```python
from build123d import *

# Parameters (mm, degrees)
F1_DEPTH         = 844.55
F3_D             = 4.7625
F3_DEPTH         = 25.4
F3_CSINK_D       = 9.525
F3_CSINK_ANGLE   = 90
F3_TIP           = 1.4307993491
F3_COPIES2_COUNT = 2


# Not quite as in the source:
# - a pattern or mirror of a feature is missing from the dataset's text; its kind, count and spacing are read off the source's solid


with BuildPart() as f1:
    # F0 (on Front) → F1 (new body, symmetric)
    with BuildSketch(Plane.XZ):
        Polygon((155.575, -103.1875), (155.575, 103.1875), (-155.575, 103.1875), (-155.575, -103.1875), (-152.4, -103.1875), (-152.4, 100.0125), (152.4, 100.0125), (152.4, -103.1875), align=None)
    extrude(amount=F1_DEPTH, both=True)

    # F3
    with Locations(Plane.YZ.offset(155.575)):
        with Locations((-793.75, -52.3875)):
            f3 = CounterSinkHole(F3_D / 2, F3_CSINK_D / 2, depth=F3_DEPTH, counter_sink_angle=F3_CSINK_ANGLE)
            with Locations((0, 0, -(F3_DEPTH + F3_TIP / 2))):  # 118° drill point
                Cone(0, F3_D / 2, F3_TIP, mode=Mode.SUBTRACT)

    # F3_copies: F3 across plane
    add(f3.mirror(Plane(origin=(0, 0, 0), x_dir=(0, 0, -1), z_dir=(-1, 0, 0))), mode=Mode.SUBTRACT)

    # F3_copies1: F3 across plane
    add(f3.mirror(Plane.ZX), mode=Mode.SUBTRACT)

    # F3_copies2: F3 ×2 about axis
    f3_copies2_axis = Axis((0, 0, 0), (0, 0, 1))
    for i in range(1, F3_COPIES2_COUNT):
        add(f3.rotate(f3_copies2_axis, i * 360 / F3_COPIES2_COUNT), mode=Mode.SUBTRACT)


solid = f1.part
```
Could you check a few things on this model? Use its own coordinates, in mm. A direction names the side the tool comes from. Round coordinates to 2 decimals unless told otherwise and drop trailing zeros. Loops run counter-clockwise (first coordinate to the right, second up) from the corner with the lowest first, then second, coordinate; pieces in that order, holes last. Notation, with made-up numbers: (12, 78) - (63, 78) arc R13 cw to (63, 97) - close; hole circle Ø9 at (-5, 86.25). An arc over 180 degrees is marked (long way). Answer in a Markdown table with one row per item. Add a question column.
(1) For faces 1 (the face through (-2, -12, 100.012)), 2 (the face through (2, -12, 103.188)), which set-ups out of +Z, -Z, +X, -X, +Y, -Y let a thin tool reach every point of the face, with its end or its side?
(2) I'm going to push flat-ended pins straight in: pin 1 (1.5 mm diameter, centred on x = 100.5, y = 98.5, fed in from -Z); pin 2 (5.5 mm diameter, centred on y = -793.75, z = -52.39, fed in from +X) (3 decimals); pin 3 (5.5 mm diameter, centred on y = -793.75, z = -52.39, fed in from -X) (3 decimals). Where does each tip first touch, or does it pass through?
(3) If we section it at A-A (z = 50.5): Please give me the cut outline in (x, y) (3 decimals), plus the area to 3 significant figures.
(4) I need wall thicknesses on line 1 along X through (y, z) = (349.5, -20.5) (3 decimals); line 2 along Z through (x, y) = (-153, 793); line 3 along Z through (x, y) = (81, 38). Which ranges of each line are inside material? Lowest first, please.
(5) If we section it at C-C (x = 69.5): Please give me the cut outline in (y, z), plus the area to 3 significant figures.
(6) If we mould it in two halves opening along X, with no side actions, what happens to faces 3 (the face through (155.575, -12, -1)), 4 (the face through (152.4, -12, 0)), 5 (the face through (-155.575, -12, 1)), 6 (the face through (-152.4, -12, -3))? For each: pulls with the +X half, pulls with the -X half, needs draft (parallel to the pull), parting line crosses it, or undercut.
(7) If we section it at B-B (y = -333): Please give me the cut outline in (x, z) (1 decimal).
Model answer:
| question | item | result |
|---|---|---|
| 1 | face 1 | -Z, +Y, -Y |
| 1 | face 2 | +Z, +X, -X, +Y, -Y |
| 2 | pin 1 | stops at z = 100.01 |
| 2 | pin 2 | stops at x = 153.565 |
| 2 | pin 3 | stops at x = -153.565 |
| 3 | outline | (-155.575, -844.55) - (-152.4, -844.55) - (-152.4, 844.55) - (-155.575, 844.55) - close; (152.4, -844.55) - (155.575, -844.55) - (155.575, 844.55) - (152.4, 844.55) - close |
| 3 | area | 10,700 mm² |
| 4 | line 1 | x = -155.575 to -152.4, 152.4 to 155.575 |
| 4 | line 2 | z = -103.19 to -54.65, -50.13 to 103.19 |
| 4 | line 3 | z = 100.01 to 103.19 |
| 5 | outline | (-844.55, 100.01) - (844.55, 100.01) - (844.55, 103.19) - (-844.55, 103.19) - close |
| 5 | area | 5,360 mm² |
| 6 | face 3 | pulls with the +X half |
| 6 | face 4 | undercut |
| 6 | face 5 | pulls with the -X half |
| 6 | face 6 | undercut |
| 7 | outline | (-155.6, -103.2) - (-152.4, -103.2) - (-152.4, 100) - (152.4, 100) - (152.4, -103.2) - (155.6, -103.2) - (155.6, 103.2) - (-155.6, 103.2) - close |
